from build123d import *

# Parameters (mm, degrees)
BOSS_EXTRUDE1_DEPTH = 8.5
SKETCH2_R           = 1
CUT_EXTRUDE1_DEPTH  = 2
FILLET1_R           = 0.2


with BuildPart() as part:
    # Sketch1 → Boss-Extrude1 (new, symmetric)
    with BuildSketch(Plane.XY):
        with BuildLine():
            Line((2.5, 0), (6, 0))
            Line((6, 0), (6, 5))
            Line((6, 5), (-6, 5))
            Line((-6, 5), (-6, 0))
            Line((-6, 0), (-2.5, 0))
            Line((-2.5, 0), (-2.5, 1.2))
            ThreePointArc((-2.5, 1.2), (-2.25, 1.45), (-2.5, 1.7))
            Line((-2.5, 1.7), (-2.5, 2.7))
            Line((-2.5, 2.7), (2.5, 2.7))
            Line((2.5, 2.7), (2.5, 1.7))
            ThreePointArc((2.5, 1.7), (2.25, 1.45), (2.5, 1.2))
            Line((2.5, 1.2), (2.5, 0))
        make_face()
    extrude(amount=BOSS_EXTRUDE1_DEPTH, both=True)

    # Sketch2 → Cut-Extrude1 (cut)
    with BuildSketch(Plane(origin=(0, 5, 0), x_dir=(1, 0, 0), z_dir=(0, 1, 0))):
        with Locations(Location((4, 0, 0), (0, 0, 270))):
            Circle(SKETCH2_R)
        with Locations(Location((-4, 0, 0), (0, 0, 90))):
            Circle(SKETCH2_R)
    extrude(amount=-CUT_EXTRUDE1_DEPTH, mode=Mode.SUBTRACT)

    # Fillet1
    fillet1_edges = [part.edges().sort_by_distance(p)[0] for p in [
        (-6, 5, 0),
        (6, 5, 0),
    ]]
    fillet(fillet1_edges, radius=FILLET1_R)


solid = part.part
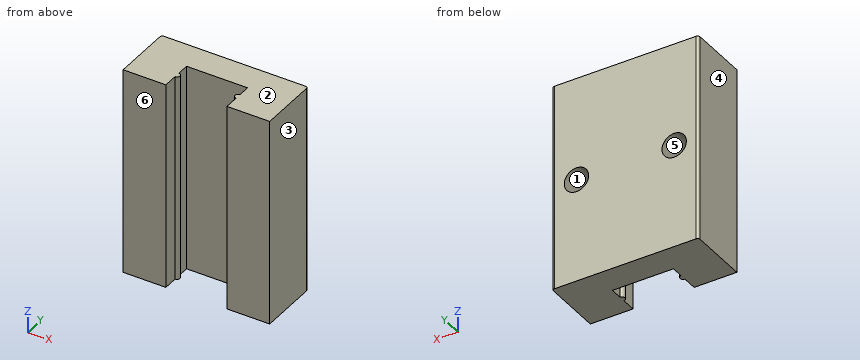
Could you check a few things on this model? Use its own coordinates, in mm. Face numbers are marked on the shaded views. A direction names the side the tool comes from. Round coordinates to 2 decimals unless told otherwise and drop trailing zeros. Order: outer loops, then holes, each group sorted by start corner. A loop starts at its lowest first (then second) coordinate and runs counter-clockwise, first axis right, second up. Notation, with made-up numbers: M 37,43 L 67,43 A28 cw 67,62 Z; hole C 18,-4 d5. An arc over 180 degrees is marked long. One line per item, written item: value.
(1) Imagine slicing it at D-D (y = 3.55). Write out the boundary of the cut face in (x, z), and give its area (3 significant figures).
Ans:
outline: M -6,-8.5 L 6,-8.5 L 6,8.5 L -6,8.5 Z; hole C -4,0 d2; hole C 4,0 d2
area: 198 mm^2
(2) I need wall thicknesses on line 1 along X through (y, z) = (4.05, 0); line 2 along X through (y, z) = (0.4, -2.75); line 3 along Z through (x, y) = (-4, 3.6). Which ranges of each line are inside material? Lowest first, please. Write a range as from..to.
Ans:
line 1: x = -6..-5, -3..3, 5..6
line 2: x = -6..-2.5, 2.5..6
line 3: z = -8.5..-1, 1..8.5
(3) Imagine slicing it at B-B (x = 4). Write out the boundary of the cut face in (y, z).
Ans:
outline: M 0,-8.5 L 5,-8.5 L 5,-1 L 3,-1 L 3,1 L 5,1 L 5,8.5 L 0,8.5 Z
(4) Imagine slicing it at C-C (z = 0). Write out the boundary of the cut face in (x, y), and give its area (3 significant figures).
Ans:
outline: M -6,0 L -2.5,0 L -2.5,1.2 A0.25 ccw -2.5,1.7 L -2.5,2.7 L 2.5,2.7 L 2.5,1.7 A0.25 ccw 2.5,1.2 L 2.5,0 L 6,0 L 6,4.8 A0.2 ccw 5.8,5 L 5,5 L 5,3 L 3,3 L 3,5 L -3,5 L -3,3 L -5,3 L -5,5 L -5.8,5 A0.2 ccw -6,4.8 Z
area: 38.7 mm^2
(5) Which directions (+Z, -Z, +X, -X, +Y, -Y) give clear straight access to the entire face, cutting with the end or side of a thin tool? Please do the marked faces 5 and 6.
Ans:
face 5: +Y
face 6: +Z, -Z, +X, -X, -Y
(6) Imagine slicing it at A-A (y = 1.45). Write out the boundary of the cut face in (x, z), and give its area (4 significant figures).
Ans:
outline: M -6,-8.5 L -2.25,-8.5 L -2.25,8.5 L -6,8.5 Z; M 2.25,-8.5 L 6,-8.5 L 6,8.5 L 2.25,8.5 Z
area: 127.5 mm^2
(7) I'm going to push a flat-ended pin straight in: P1, Ø1.8, axis at x = -4, z = 0, coming from the +Y side. Where does the tip first touch, or does it pass through?
Ans:
P1: stops at y = 3
(8) If we mould it in two halves opening along X, with no side actions, what happens to the marked faces 1, 2, 3 and 4? For each: released by +X, released by -X, zero draft, split by the parting line, or undercut.
Ans:
face 1: undercut
face 2: zero draft
face 3: released by +X
face 4: released by -X
